Design review of the part built by this model. Coordinates are the model's own, in mm. A direction names the side the tool comes from. Round coordinates to 2 decimals unless told otherwise and drop trailing zeros. Loops run counter-clockwise (first coordinate to the right, second up) from the corner with the lowest first, then second, coordinate; pieces in that order, holes last. Notation, with made-up numbers: (-4, 86) - (42, 86) arc R26 cw to (42, 114) - close; hole circle Ø5 at (-23, -39). An arc over 180 degrees is marked (long way). Return JSON: item names as keys, results as strings. Group by question number.
(1) We need section D-D, the plane z = -40.5. Write out the cut boundary in (x, y).
(2) We need section B-B, the plane y = 28.5. Write out the cut boundary in (x, z).
(3) We need section C-C, the plane x = 9.5. Write out the cut boundary in (y, z), and give its area (3 significant figures).
(4) The part is to be moulded in two halves that separate along Z. For faces 3 (the flat face through (48, 1, -3)), 4 (the flat face through (1, 25, -38.25)), 5 (the flat face through (13.5, 0, -25.4)), say which applies: pulls with the +Z half, pulls with the -Z half, needs draft (parallel to the pull), parting line crosses it, or undercut.
(5) Clearance check with flat-ended pins moving along their axes: pin 1 (1.5 mm diameter, centred on y = 28.5, z = -36.5, fed in from +X); pin 2 (2 mm diameter, centred on x = 38.5, z = -31, fed in from +Y). State where each tip first meets the part, or that it passes through.
(6) For faces 1 (the flat face through (50, 1, -25)), 2 (the flat face through (1, 25, -11.75)), list the 3-axis set-ups (+Z, -Z, +X, -X, +Y, -Y) from which the entire face can be reached by the end or side of a thin tool; tool diameter is ignored.
(7) Wall thickness on L1, parallel to X at y = 0.85, z = -9.5; L2, parallel to Z at x = 40, y = 2; L3, parallel to Y at x = 46, z = -33.5: over which ranges is each line inside the solid? List them lowest first. Write a range as [from, to].
(8) We need section A-A, the plane z = -25. Write out the cut boundary in (x, y).
from build123d import *

# Parameters (mm, degrees)
SKETCH1_W           = 50
SKETCH1_H           = 50
SKETCH1_R           = 11
SKETCH1_R_2         = 1.75
BOSS_EXTRUDE1_DEPTH = 3
SKETCH2_W           = 3
SKETCH2_H           = 50
BOSS_EXTRUDE2_DEPTH = 47
CUT_EXTRUDE1_REACH  = 88.603
CHAMFER1_SIZE       = 5
CHAMFER2_SIZE       = 5


with BuildPart() as part:
    # Sketch1 → Boss-Extrude1 (new body)
    with BuildSketch(Plane(origin=(0, 0, 0), x_dir=(1, 0, 0), z_dir=(0, 1, 0))):
        with Locations((25, 25)):
            Rectangle(SKETCH1_W, SKETCH1_H)
        with Locations(Location((25, 25, 0), (0, 0, 270))):
            Circle(SKETCH1_R, mode=Mode.SUBTRACT)
        with Locations(Location((40.5, 40.5, 0), (0, 0, 270))):
            Circle(SKETCH1_R_2, mode=Mode.SUBTRACT)
        with Locations(Location((9.5, 40.5, 0), (0, 0, 270))):
            Circle(SKETCH1_R_2, mode=Mode.SUBTRACT)
        with Locations(Location((9.5, 9.5, 0), (0, 0, 270))):
            Circle(SKETCH1_R_2, mode=Mode.SUBTRACT)
        with Locations(Location((40.5, 9.5, 0), (0, 0, 270))):
            Circle(SKETCH1_R_2, mode=Mode.SUBTRACT)
    extrude(amount=BOSS_EXTRUDE1_DEPTH)

    # Sketch2 → Boss-Extrude2 (add)
    with BuildSketch(Plane(origin=(0, 3, 0), x_dir=(1, 0, 0), z_dir=(0, 1, 0))):
        with Locations((1.5, 25)):
            Rectangle(SKETCH2_W, SKETCH2_H)
    extrude(amount=BOSS_EXTRUDE2_DEPTH)

    # Sketch3 → Cut-Extrude1 (cut, up to next)
    with BuildSketch(Plane.ZY, mode=Mode.PRIVATE) as cut_extrude1_sk1:
        with BuildLine():
            Line((-38.25, 42), (-38.25, 8))
            ThreePointArc((-38.25, 8), (-40, 6.25), (-41.75, 8))
            Line((-41.75, 8), (-41.75, 42))
            ThreePointArc((-41.75, 42), (-40, 43.75), (-38.25, 42))
        make_face()
    cut_extrude1_tool1 = extrude(cut_extrude1_sk1.sketch, amount=-CUT_EXTRUDE1_REACH, mode=Mode.PRIVATE) & part.part
    # Sketch3 → Cut-Extrude1 (cut, up to next)
    with BuildSketch(Plane.ZY, mode=Mode.PRIVATE) as cut_extrude1_sk2:
        with BuildLine():
            Line((-11.75, 42), (-11.75, 8))
            ThreePointArc((-11.75, 8), (-10, 6.25), (-8.25, 8))
            Line((-8.25, 8), (-8.25, 42))
            ThreePointArc((-8.25, 42), (-10, 43.75), (-11.75, 42))
        make_face()
    cut_extrude1_tool2 = extrude(cut_extrude1_sk2.sketch, amount=-CUT_EXTRUDE1_REACH, mode=Mode.PRIVATE) & part.part
    add(cut_extrude1_tool1.solids().sort_by_distance((0, 25, -40))[0], mode=Mode.SUBTRACT)
    add(cut_extrude1_tool2.solids().sort_by_distance((0, 25, -10))[0], mode=Mode.SUBTRACT)

    # Chamfer1
    chamfer1_edges = [part.edges().sort_by_distance(p)[0] for p in [
        (1.5, 50, 0),
        (1.5, 50, -50),
    ]]
    chamfer(chamfer1_edges, length=CHAMFER1_SIZE)

    # Chamfer2
    chamfer2_edges = [part.edges().sort_by_distance(p)[0] for p in [
        (50, 1.5, -50),
        (50, 1.5, 0),
    ]]
    chamfer(chamfer2_edges, length=CHAMFER2_SIZE)


solid = part.part
Solutions:
{
 "1": {"outline": "(0, 0) - (7.75, 0) - (7.75, 3) - (3, 3) - (3, 6.32) - (0, 6.32) - close; (0, 43.68) - (3, 43.68) - (3, 50) - (0, 50) - close; (11.25, 0) - (38.75, 0) - (38.75, 3) - (11.25, 3) - close; (42.25, 0) - (50, 0) - (50, 3) - (42.25, 3) - close"},
 "2": {"outline": "(0, -50) - (3, -50) - (3, -41.75) - (0, -41.75) - close; (0, -38.25) - (3, -38.25) - (3, -11.75) - (0, -11.75) - close; (0, -8.25) - (3, -8.25) - (3, 0) - (0, 0) - close"},
 "3": {"outline": "(0, -50) - (3, -50) - (3, -42.25) - (0, -42.25) - close; (0, -38.75) - (3, -38.75) - (3, -11.25) - (0, -11.25) - close; (0, -7.75) - (3, -7.75) - (3, 0) - (0, 0) - close", "area": "129 mm^2"},
 "4": {"face 3": "pulls with the +Z half", "face 4": "undercut", "face 5": "needs draft"},
 "5": {"pin 1": "x = 3", "pin 2": "y = 3"},
 "6": {"face 1": "+Z, -Z, +X, +Y, -Y", "face 2": "+X, -X"},
 "7": {"L1": "[0, 7.75], [11.25, 38.75], [42.25, 50]", "L2": "[-50, -42.18], [-38.82, -11.18], [-7.82, 0]", "L3": "[0, 3]"},
 "8": {"outline": "(0, 0) - (14, 0) - (14, 3) - (3, 3) - (3, 50) - (0, 50) - close; (36, 0) - (50, 0) - (50, 3) - (36, 3) - close"}
}
